```python
from build123d import *

# Parameters (mm, degrees)
SKETCH1_W          = 5
SKETCH1_H          = 5
SKETCH1_W_2        = 10
REVOLVE1_ANGLE     = 270
CUT_REVOLVE1_START = 5
CUT_REVOLVE1_DEPTH = 10


# Read off the part's stored shape, not the designer's step: Cut-Revolve1
with BuildPart() as part:
    # Sketch1 → Revolve1 (revolve)
    with BuildSketch(Plane.XY):
        with Locations((2.5, -2.5)):
            Rectangle(SKETCH1_W, SKETCH1_H)
        with Locations((17.5, -2.5)):
            Rectangle(SKETCH1_W, SKETCH1_H)
        with Locations((10, -2.5)):
            Rectangle(SKETCH1_W_2, SKETCH1_H)
    revolve(axis=Axis((-365.597578267, 25, 0), (1, 0, 0)), revolution_arc=REVOLVE1_ANGLE)

    # Cut-Revolve1 outline → Cut-Revolve1 (cut)
    with BuildSketch(Plane.YZ.offset(CUT_REVOLVE1_START)):
        with BuildLine():
            Line((10, -25.980762114), (12.5, -21.650635095))
            ThreePointArc((12.5, -21.650635095), (3.349364905, -12.5), (0, 0))
            Line((0, 0), (-5, 0))
            ThreePointArc((-5, 0), (-0.980762114, -15), (10, -25.980762114))
        make_face()
    extrude(amount=CUT_REVOLVE1_DEPTH, mode=Mode.SUBTRACT)


solid = part.part
```
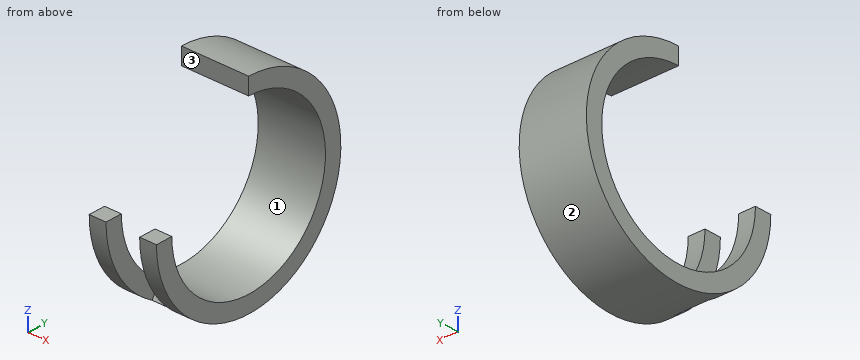
Input: part model. Units: mm. Frame: model coordinates. Face numbers are marked on the shaded views. Give positions to 0.01 mm unless a question says otherwise; leave off trailing zeros. Loops run counter-clockwise (first coordinate to the right, second up) from the corner with the lowest first, then second, coordinate; pieces in that order, holes last. Notation, with made-up numbers: (38.5, 33) -> (42.5, 33) arc R35 cw to (42.5, 72) -> close; hole circle Ø11 at (-37, -1.75). An arc over 180 degrees is marked (long way). Use a Markdown table: item, result.
Q1. Section query D-D, the plane x = 12.75. Return the cut outline in (y, z), plus the area to 3 significant figures.
Entries:
| item | result |
|---|---|
| outline | (10, -25.98) arc R30 ccw (long way) to (25, 30) -> (25, 25) arc R25 cw (long way) to (12.5, -21.65) -> close |
| area | 504 mm² |
Q2. First-contact query: P1, Ø8, axis at x = 15.5, y = 39.5, coming from the +Z side; P2, Ø1.5, axis at x = 2.5, y = 21.5, coming from the +Z side; P3, Ø8, axis at x = 3, z = 13, coming from the -Y side; P4, Ø2, axis at y = 12.5, z = -20, coming from the +X side. Flat tips, straight axial feed; report the tip coordinate or a pass-through.
Entries:
| item | result |
|---|---|
| P1 | stops at z = 28.1 |
| P2 | stops at z = -24.64 |
| P3 | stops at y = 43.33 |
| P4 | passes through |
Q3. Ray query, probe 1 along Y at (x, z) = (7, 0); probe 2 along Y at (x, z) = (10, -22); probe 3 along Y at (x, z) = (3.75, -21). Return the intervals inside material, ascending. Write a range as from..to.
Entries:
| item | result |
|---|---|
| probe 1 | y = 50..55 |
| probe 2 | y = 12.3..13.13, 36.87..45.4 |
| probe 3 | y = 3.58..11.44, 38.56..46.42 |
Q4. Section query C-C, the plane y = 37.5. Return the cut outline in (x, z), plus the area to 3 significant figures.
Entries:
| item | result |
|---|---|
| outline | (0, -27.27) -> (20, -27.27) -> (20, -21.65) -> (0, -21.65) -> close; (0, 21.65) -> (20, 21.65) -> (20, 27.27) -> (0, 27.27) -> close |
| area | 225 mm² |
Q5. Section query A-A, the plane z = -23.5. Return the cut outline in (x, y).
Entries:
| item | result |
|---|---|
| outline | (0, 6.35) -> (5, 6.35) -> (5, 11.43) -> (15, 11.43) -> (15, 6.35) -> (20, 6.35) -> (20, 16.47) -> (0, 16.47) -> close; (0, 33.53) -> (20, 33.53) -> (20, 43.65) -> (0, 43.65) -> close |
Q6. Pull-direction query (Z, two-part tool) for the marked faces 1, 2 and 3; classes: pulls with the +Z half, pulls with the -Z half, needs draft (parallel to the pull), parting line crosses it, or undercut.
Entries:
| item | result |
|---|---|
| face 1 | undercut |
| face 2 | parting line crosses it |
| face 3 | needs draft |
Q7. Section query B-B, the plane z = -3. Return the cut outline in (x, y).
Entries:
| item | result |
|---|---|
| outline | (0, -4.85) -> (5, -4.85) -> (5, 0.18) -> (0, 0.18) -> close; (0, 49.82) -> (20, 49.82) -> (20, 54.85) -> (0, 54.85) -> close; (15, -4.85) -> (20, -4.85) -> (20, 0.18) -> (15, 0.18) -> close |
